CAD build for the part. Positions are in the model's coordinates, mm. A direction names the side the tool comes from. Coordinates: 2 decimals unless noted, no trailing zeros. Write each loop counter-clockwise with the first axis right and the second up, starting at its lowest first coordinate (ties: lowest second). Pieces come first, ordered by that corner, then holes. Notation, with made-up numbers: (-10, 72) -> (1, 72) arc R15 ccw to (1, 80) -> close; hole circle Ø8 at (16, 80). An arc over 180 degrees is marked (long way). Answer as CSV lines item,"result".
```python
from build123d import *

# Parameters (mm, degrees)
SKETCH1_W           = 28.5
SKETCH1_H           = 28.5
BOSS_EXTRUDE1_DEPTH = 7
FILLET1_R           = 2
SKETCH2_R           = 11
BOSS_EXTRUDE2_DEPTH = 1.6
SKETCH3_R           = 4
CUT_EXTRUDE1_DEPTH  = 1.6
SKETCH4_R           = 2.5
BOSS_EXTRUDE3_DEPTH = 20
SKETCH5_W           = 4.4
SKETCH5_H           = 1
CUT_EXTRUDE2_DEPTH  = 20
SKETCH6_W           = 28.2
SKETCH6_H           = 28.2
BOSS_EXTRUDE4_DEPTH = 14
FILLET2_R           = 2
SKETCH7_W           = 28.5
SKETCH7_H           = 28.5
BOSS_EXTRUDE5_DEPTH = 7
FILLET3_R           = 2
SKETCH8_W           = 15
SKETCH8_H           = 5
BOSS_EXTRUDE6_DEPTH = 2.7
SKETCH9_R           = 1.4
CUT_EXTRUDE3_DEPTH  = 42.7
SKETCH10_R          = 3.5
CUT_EXTRUDE4_DEPTH  = 4
FILLET4_R           = 0.5
FILLET5_R           = 0.5
CUT_EXTRUDE5_START  = -0.1
SKETCH11_R          = 12
SKETCH11_R_2        = 11
CUT_EXTRUDE5_DEPTH  = 0.1
CUT_EXTRUDE6_START  = -2.5
SKETCH12_R          = 4
CUT_EXTRUDE6_DEPTH  = 2.5
BOSS_EXTRUDE7_START = 0.5
SKETCH13_R          = 2.5
BOSS_EXTRUDE7_DEPTH = 0.5
FILLET6_R           = 0.2
SKETCH14_W          = 1
SKETCH14_H          = 1
CUT_EXTRUDE7_DEPTH  = 5


with BuildPart() as part:
    # Sketch1 → Boss-Extrude1 (new body)
    with BuildSketch(Plane.XY):
        Rectangle(SKETCH1_W, SKETCH1_H)
    extrude(amount=BOSS_EXTRUDE1_DEPTH)

    # Fillet1
    fillet1_edges = [part.edges().sort_by_distance(p)[0] for p in [
        (14.25, -14.25, 3.5),
        (-14.25, -14.25, 3.5),
        (-14.25, 14.25, 3.5),
        (14.25, 14.25, 3.5),
    ]]
    fillet(fillet1_edges, radius=FILLET1_R)

    # Sketch2 → Boss-Extrude2 (add)
    with BuildSketch(Plane.XY.offset(7)):
        Circle(SKETCH2_R)
    extrude(amount=BOSS_EXTRUDE2_DEPTH)

    # Sketch3 → Cut-Extrude1 (cut)
    with BuildSketch(Plane.XY.offset(8.6)):
        Circle(SKETCH3_R)
    extrude(amount=-CUT_EXTRUDE1_DEPTH, mode=Mode.SUBTRACT)

    # Sketch4 → Boss-Extrude3 (add)
    with BuildSketch(Plane.XY.offset(7)):
        Circle(SKETCH4_R)
    extrude(amount=BOSS_EXTRUDE3_DEPTH)

    # Sketch5 → Cut-Extrude2 (cut)
    with BuildSketch(Plane.XY.offset(27)):
        with Locations((0, 2.5)):
            Rectangle(SKETCH5_W, SKETCH5_H)
    extrude(amount=-CUT_EXTRUDE2_DEPTH, mode=Mode.SUBTRACT)

    # Sketch6 → Boss-Extrude4 (add)
    with BuildSketch(Plane(origin=(0, 0, 0), x_dir=(-1, 0, 0), z_dir=(0, 0, -1))):
        Rectangle(SKETCH6_W, SKETCH6_H)
    extrude(amount=BOSS_EXTRUDE4_DEPTH)

    # Fillet2
    # the kernel refuses this fillet: 2 mm, written as the material it takes off along each edge
    with BuildSketch(Plane(origin=(-14.1, -14.1, 0), x_dir=(0, 1, 0), z_dir=(0, 0, -1)), Plane(origin=(-14.1, 14.1, 0), x_dir=(1, 0, 0), z_dir=(0, 0, -1))) as fillet2_piece_1:
        with BuildLine():
            CenterArc((FILLET2_R, FILLET2_R), FILLET2_R, 180, 90)
            Line((0, FILLET2_R), (0, 0))
            Line((0, 0), (FILLET2_R, 0))
        make_face()
    extrude(amount=19, mode=Mode.SUBTRACT)
    with BuildSketch(Plane(origin=(14.1, 14.1, 0), x_dir=(-1, 0, 0), z_dir=(0, 0, -1)), Plane(origin=(14.1, -14.1, 0), x_dir=(0, 1, 0), z_dir=(0, 0, -1))) as fillet2_piece_2:
        with BuildLine():
            CenterArc((FILLET2_R, -FILLET2_R), FILLET2_R, 90, 90)
            Line((0, -FILLET2_R), (0, 0))
            Line((0, 0), (FILLET2_R, 0))
        make_face()
    extrude(amount=19, mode=Mode.SUBTRACT)

    # Sketch7 → Boss-Extrude5 (add)
    with BuildSketch(Plane(origin=(0, 0, -14), x_dir=(-1, 0, 0), z_dir=(0, 0, -1))):
        Rectangle(SKETCH7_W, SKETCH7_H)
    extrude(amount=BOSS_EXTRUDE5_DEPTH)

    # Fillet3
    fillet3_edges = [part.edges().sort_by_distance(p)[0] for p in [
        (-14.25, -14.25, -17.5),
        (-14.25, 14.25, -17.5),
        (14.25, 14.25, -17.5),
        (14.25, -14.25, -17.5),
    ]]
    fillet(fillet3_edges, radius=FILLET3_R)

    # Sketch8 → Boss-Extrude6 (add)
    with BuildSketch(Plane(origin=(0, 14.25, 0), x_dir=(1, 0, 0), z_dir=(0, 1, 0))):
        with Locations((0, 17)):
            Rectangle(SKETCH8_W, SKETCH8_H)
    extrude(amount=BOSS_EXTRUDE6_DEPTH)

    # Sketch9 → Cut-Extrude3 (cut)
    with BuildSketch(Plane.XY.offset(7)):
        with Locations((-11.5, 11.5)):
            Circle(SKETCH9_R)
        with Locations((11.5, 11.5)):
            Circle(SKETCH9_R)
        with Locations((11.5, -11.5)):
            Circle(SKETCH9_R)
        with Locations((-11.5, -11.5)):
            Circle(SKETCH9_R)
    extrude(amount=-CUT_EXTRUDE3_DEPTH, mode=Mode.SUBTRACT)

    # Sketch10 → Cut-Extrude4 (cut)
    with BuildSketch(Plane(origin=(0, 0, -21), x_dir=(-1, 0, 0), z_dir=(0, 0, -1))):
        with Locations((-11.5, 11.5)):
            Circle(SKETCH10_R)
        with Locations((11.5, 11.5)):
            Circle(SKETCH10_R)
        with Locations((11.5, -11.5)):
            Circle(SKETCH10_R)
        with Locations((-11.5, -11.5)):
            Circle(SKETCH10_R)
    extrude(amount=-CUT_EXTRUDE4_DEPTH, mode=Mode.SUBTRACT)

    # Fillet4
    fillet4_edges = [part.edges().sort_by_distance(p)[0] for p in [
        (14.25, -9.334936491, -19),
        (9.334936491, -14.25, -19),
        (-14.25, -9.334936491, -19),
        (-9.334936491, -14.25, -19),
        (-9.334936491, 14.25, -19),
        (-14.25, 9.334936491, -19),
        (9.334936491, 14.25, -19),
        (14.25, 9.334936491, -19),
    ]]
    fillet(fillet4_edges, radius=FILLET4_R)

    # Fillet5
    fillet5_edges = [part.edges().sort_by_distance(p)[0] for p in [
        (-14.25, 0, -21),
        (9.025126266, -9.025126266, -21),
        (0, -14.25, -21),
        (-9.025126266, -9.025126266, -21),
        (-9.025126266, 9.025126266, -21),
        (0, 14.25, -21),
        (9.025126266, 9.025126266, -21),
        (14.25, 0, -21),
        (13.983853587, 8.634752599, -21),
        (8.634752599, 13.983853587, -21),
        (13.983853587, -8.634752599, -21),
        (8.634752599, -13.983853587, -21),
        (-8.634752599, -13.983853587, -21),
        (-13.983853587, -8.634752599, -21),
        (-8.634752599, 13.983853587, -21),
        (-13.983853587, 8.634752599, -21),
    ]]
    fillet(fillet5_edges, radius=FILLET5_R)

    # Sketch11 → Cut-Extrude5 (cut)
    with BuildSketch(Plane.XY.offset(7).offset(CUT_EXTRUDE5_START)):
        Circle(SKETCH11_R)
        Circle(SKETCH11_R_2, mode=Mode.SUBTRACT)
    extrude(amount=CUT_EXTRUDE5_DEPTH, mode=Mode.SUBTRACT)

    # Sketch12 → Cut-Extrude6 (cut)
    with BuildSketch(Plane(origin=(0, 0, -21), x_dir=(-1, 0, 0), z_dir=(0, 0, -1)).offset(CUT_EXTRUDE6_START)):
        with Locations(Location((0, 0, 0), (0, 0, 180))):
            Circle(SKETCH12_R)
    extrude(amount=CUT_EXTRUDE6_DEPTH, mode=Mode.SUBTRACT)

    # Sketch13 → Boss-Extrude7 (add)
    with BuildSketch(Plane(origin=(0, 0, -18.5), x_dir=(-1, 0, 0), z_dir=(0, 0, -1)).offset(BOSS_EXTRUDE7_START)):
        Circle(SKETCH13_R)
    extrude(amount=-BOSS_EXTRUDE7_DEPTH)

    # Fillet6
    fillet6_edges = [part.edges().sort_by_distance(p)[0] for p in [
        (2.5, 0, -19),
    ]]
    fillet(fillet6_edges, radius=FILLET6_R)

    # Sketch14 → Cut-Extrude7 (cut)
    with BuildSketch(Plane(origin=(0, 16.95, 0), x_dir=(1, 0, 0), z_dir=(0, 1, 0))):
        with Locations((-6.3, 17)):
            Rectangle(SKETCH14_W, SKETCH14_H)
        with Locations((-3.76, 17)):
            Rectangle(SKETCH14_W, SKETCH14_H)
        with Locations((-1.22, 17)):
            Rectangle(SKETCH14_W, SKETCH14_H)
        with Locations((1.32, 17)):
            Rectangle(SKETCH14_W, SKETCH14_H)
        with Locations((3.86, 17)):
            Rectangle(SKETCH14_W, SKETCH14_H)
        with Locations((6.4, 17)):
            Rectangle(SKETCH14_W, SKETCH14_H)
    extrude(amount=-CUT_EXTRUDE7_DEPTH, mode=Mode.SUBTRACT)


solid = part.part
```
Item 1: 3-axis set-ups, long thin cutter, end or side, ignore diameter. For faces 1 (the flat face through (14.1, 0, -7)), 2 (the cylindrical face through (-13.5, -13.53, -6.9)), 3 (the flat face through (-4.26, 14, -17)), 4 (the cylindrical face through (-0.867, -3.905, 7.811)): which of +Z, -Z, +X, -X, +Y, -Y reach the whole face in a straight line?
Answer below:
face 1,"+X, +Y, -Y"
face 2,"-X, -Y"
face 3,"+Y"
face 4,"+Z"
Item 2: Saw through at C-C on y = -5.5. Give the cut face in (x, z).
Answer below:
outline,"(-14.25, -20.5) arc R0.5 ccw to (-13.75, -21) -> (13.75, -21) arc R0.5 ccw to (14.25, -20.5) -> (14.25, -14) -> (14.1, -14) -> (14.1, 0) -> (14.25, 0) -> (14.25, 7) -> (10.67, 7) -> (10.67, 6.9) -> (9.53, 6.9) -> (9.53, 8.6) -> (-9.53, 8.6) -> (-9.53, 6.9) -> (-10.67, 6.9) -> (-10.67, 7) -> (-14.25, 7) -> (-14.25, 0) -> (-14.1, 0) -> (-14.1, -14) -> (-14.25, -14) -> close"
Item 3: Wall check: line 1 (Y direction, x = 11.5, z = -10.25); line 2 (Y direction, x = 11.5, z = 0.5); line 3 (Y direction, x = 0, z = -19.05). Give the ranges that are in metal, low to high. Write a range as from..to.
Answer below:
line 1,"y = -14.1..-12.9, -10.1..10.1, 12.9..14.1"
line 2,"y = -14.25..-12.9, -10.1..10.1, 12.9..14.25"
line 3,"y = -14.25..-4, 4..16.95"
Item 4: Flat gauge pins, fed straight in: pin 1 (4 mm diameter, centred on x = 1.5, z = -5.5, fed in from -Y); pin 2 (0.8 mm diameter, centred on y = 13.5, z = -17, fed in from +X); pin 3 (1.3 mm diameter, centred on x = 2, y = 15, fed in from -Z); pin 4 (12 mm diameter, centred on x = 10, z = 15.5, fed in from -Y). Where does each tip first touch, or does it go through?
Answer below:
pin 1,"stops at y = -14.1"
pin 2,"stops at x = 14.06"
pin 3,"stops at z = -19.5"
pin 4,"passes through"
Item 5: Two-plate mould, pull along Y, no slides. Class faces 5 (the flat face through (0, 0, -19)), 6 (the flat face through (6.4, 11.95, -17)), 7 (the cylindrical face through (-12.53, -10.55, -4.83)), 8 (the flat face through (-14.1, 0, -7)): pulls with the +Y half, pulls with the -Y half, needs draft (parallel to the pull), parting line crosses it, or undercut.
Answer below:
face 5,"undercut"
face 6,"pulls with the +Y half"
face 7,"undercut"
face 8,"needs draft"
Item 6: Saw through at B-B on z = 5. Give the cut face in (x, y).
Answer below:
outline,"(-14.25, -12.25) arc R2 ccw to (-12.25, -14.25) -> (12.25, -14.25) arc R2 ccw to (14.25, -12.25) -> (14.25, 12.25) arc R2 ccw to (12.25, 14.25) -> (-12.25, 14.25) arc R2 ccw to (-14.25, 12.25) -> close; hole circle Ø2.8 at (-11.5, -11.5); hole circle Ø2.8 at (-11.5, 11.5); hole circle Ø2.8 at (11.5, -11.5); hole circle Ø2.8 at (11.5, 11.5)"
Item 7: Saw through at A-A on z = -9.5. Give the cut face in (x, y), and give its area (3 significant figures).
Answer below:
outline,"(-14.1, -12.1) arc R2 ccw to (-12.1, -14.1) -> (12.1, -14.1) arc R2 ccw to (14.1, -12.1) -> (14.1, 12.1) arc R2 ccw to (12.1, 14.1) -> (-12.1, 14.1) arc R2 ccw to (-14.1, 12.1) -> close; hole circle Ø2.8 at (-11.5, -11.5); hole circle Ø2.8 at (-11.5, 11.5); hole circle Ø2.8 at (11.5, -11.5); hole circle Ø2.8 at (11.5, 11.5)"
area,"767 mm2"
